Check sheet for the drawn part. Datum: minimum x, y, z corner. Units: mm. A direction names the side the tool comes from. Round coordinates to 2 decimals unless told otherwise and drop trailing zeros. Write each loop counter-clockwise with the first axis right and the second up, starting at its lowest first coordinate (ties: lowest second). Pieces come first, ordered by that corner, then holes. Notation, with made-up numbers: (67.25, -8.5) - (74.25, -8.5) arc R24 cw to (74.25, 21.5) - close; hole circle Ø10 at (-34.5, 84.5). An arc over 180 degrees is marked (long way). Answer as a JSON object with one key per item and string values.
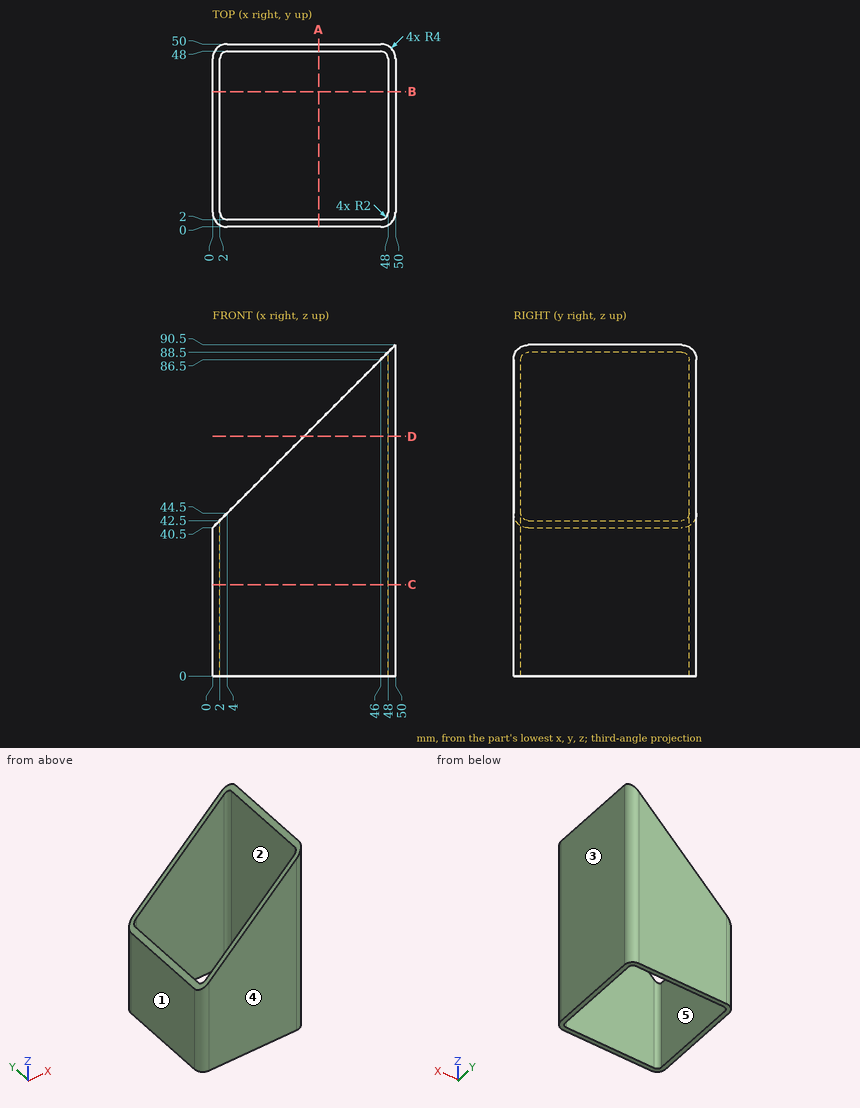
1. Go/stop test with flat-tipped pins: pin 1 (1.5 mm diameter, centred on y = 37.5, z = 54, fed in from -X); pin 2 (4 mm diameter, centred on x = 33, z = 78.5, fed in from +Y). Record where each tip stops, or that it passes through.
Completed:
{"pin 1": "stops at x = 48", "pin 2": "passes through"}
2. Access from +Z, -Z, +X, -X, +Y, -Y to the whole of each face (thin tool, end or side, straight path). Record for the marked faces 4 and 5.
Completed:
{"face 4": "+Z, -Z, +X, -X, -Y", "face 5": "+Z, -Z"}
3. Material ranges on probe 1 along Y at (x, z) = (40, 54.5); probe 2 along X at (y, z) = (23, 74), recorded low to high. Write a range as from..to.
Completed:
{"probe 1": "y = 0..2, 48..50", "probe 2": "x = 48..50"}
4. Cross-section at A-A (x = 29). Record the boundary of the cut face in (y, z), plus the area to 3 significant figures.
Completed:
{"outline": "(0, 0) - (2, 0) - (2, 69.5) - (0, 69.5) - close; (48, 0) - (50, 0) - (50, 69.5) - (48, 69.5) - close", "area": "278 mm^2"}
5. Cross-section at B-B (y = 37). Record the boundary of the cut face in (x, z).
Completed:
{"outline": "(0, 0) - (2, 0) - (2, 42.5) - (0, 40.5) - close; (48, 0) - (50, 0) - (50, 90.5) - (48, 88.5) - close"}
6. Mould release check, pull along X, two halves, no side actions. Record for the marked faces 1, 2 and 3: released by +X, released by -X, zero draft, split by the parting line, or undercut.
Completed:
{"face 1": "released by -X", "face 2": "undercut", "face 3": "released by +X"}
7. Cross-section at C-C (z = 25). Record the boundary of the cut face in (x, y), plus the area to 3 significant figures.
Completed:
{"outline": "(0, 4) arc R4 ccw to (4, 0) - (46, 0) arc R4 ccw to (50, 4) - (50, 46) arc R4 ccw to (46, 50) - (4, 50) arc R4 ccw to (0, 46) - close; hole (2, 4) arc R2 ccw to (4, 2) - (46, 2) arc R2 ccw to (48, 4) - (48, 46) arc R2 ccw to (46, 48) - (4, 48) arc R2 ccw to (2, 46) - close", "area": "374 mm^2"}
8. Cross-section at D-D (z = 65.5). Record the boundary of the cut face in (x, y).
Completed:
{"outline": "(25, 0) - (46, 0) arc R4 ccw to (50, 4) - (50, 46) arc R4 ccw to (46, 50) - (25, 50) - (25, 48) - (46, 48) arc R2 cw to (48, 46) - (48, 4) arc R2 cw to (46, 2) - (25, 2) - close"}
